Could you check a few things on this model? Use its own coordinates, in mm. A direction names the side the tool comes from. Coordinates: 2 decimals unless noted, no trailing zeros. Write each loop counter-clockwise with the first axis right and the second up, starting at its lowest first coordinate (ties: lowest second). Pieces come first, ordered by that corner, then holes.
```python
from build123d import *

# Parameters (mm, degrees)
ESBO_O1_R                = 9
ESBO_O1_R_2              = 6.15
RESSALTO_EXTRUS_O1_DEPTH = 38.8
ESBO_O1_2_R              = 6.15
RESSALTO_EXTRUS_O2_DEPTH = 41.8
ESBO_O2_R                = 1.5
CORTE_EXTRUS_O1_DEPTH    = 44.694850955


with BuildPart() as part:
    # Esbo_o1 → Ressalto-extrus_o1 (new body)
    with BuildSketch(Plane(origin=(0, 0, 0), x_dir=(1, 0, 0), z_dir=(0, 1, 0))):
        with Locations(Location((0, 0, 0), (0, 0, 270))):
            Circle(ESBO_O1_R)
        with Locations(Location((0, 0, 0), (0, 0, 270))):
            Circle(ESBO_O1_R_2, mode=Mode.SUBTRACT)
    extrude(amount=RESSALTO_EXTRUS_O1_DEPTH)

    # Esbo_o1_2 → Ressalto-extrus_o2 (add)
    with BuildSketch(Plane(origin=(0, 0, 0), x_dir=(1, 0, 0), z_dir=(0, 1, 0))):
        with Locations(Location((0, 0, 0), (0, 0, 270))):
            Circle(ESBO_O1_2_R)
    extrude(amount=RESSALTO_EXTRUS_O2_DEPTH)

    # Esbo_o2 → Corte-extrus_o1 (cut, through all)
    with BuildSketch(Plane(origin=(0, 41.8, 0), x_dir=(1, 0, 0), z_dir=(0, 1, 0))):
        with Locations(Location((0, 0, 0), (0, 0, 270))):
            Circle(ESBO_O2_R)
    extrude(amount=-CORTE_EXTRUS_O1_DEPTH, mode=Mode.SUBTRACT)


solid = part.part
```
1. For pin 1 (1 mm diameter, centred on x = -2.5, y = 31.5, fed in from -Z); pin 2 (6 mm diameter, centred on x = 6.5, y = 30, fed in from -Z); pin 3 (1.8 mm diameter, centred on x = 0, z = 0, fed in from -Y); pin 4 (2 mm diameter, centred on x = 6.5, y = 31.5, fed in from +Z), each with a flat end and sliding along its axis, tell me the tip position at first contact or that it passes through.
Verdict:
pin 1: stops at z = -8.77
pin 2: stops at z = -8.29
pin 3: passes through
pin 4: stops at z = 7.12
2. Please list where these lines run through material, in increasing order: line 1 along X through (y, z) = (24.5, 0); line 2 along Y through (x, z) = (0.25, -8); line 3 along Z through (x, y) = (-1.25, 12).
Verdict:
line 1: x = -9 to -1.5, 1.5 to 9
line 2: y = 0 to 38.8
line 3: z = -8.91 to -0.83, 0.83 to 8.91
3. I want a section at A-A on z = 0. Please give me the cut outline in (x, y), plus the area to 3 significant figures.
Verdict:
outline: (-9, 0) - (-1.5, 0) - (-1.5, 41.8) - (-6.15, 41.8) - (-6.15, 38.8) - (-9, 38.8) - close; (1.5, 0) - (9, 0) - (9, 38.8) - (6.15, 38.8) - (6.15, 41.8) - (1.5, 41.8) - close
area: 610 mm2
4. If we mould it in two halves opening along X, with no side actions, what happens to faces 3 (the face through (0.45, 21.19, 1.43)), 4 (the face through (2.703, 19.128, 8.584)), 5 (the face through (-2, 0, 0))? For each: pulls with the +X half, pulls with the -X half, needs draft (parallel to the pull), parting line crosses it, or undercut.
Verdict:
face 3: undercut
face 4: parting line crosses it
face 5: needs draft
5. I want a section at B-B on x = 0. Please give me the cut outline in (y, z).
Verdict:
outline: (0, -9) - (38.8, -9) - (38.8, -6.15) - (41.8, -6.15) - (41.8, -1.5) - (0, -1.5) - close; (0, 1.5) - (41.8, 1.5) - (41.8, 6.15) - (38.8, 6.15) - (38.8, 9) - (0, 9) - close
6. I want a section at C-C on y = 28. Please give me the cut outline in (x, z).
Verdict:
outline: circle Ø18 at (0, 0); hole circle Ø3 at (0, 0)
7. I want a section at D-D on x = -2.5. Please give me the cut outline in (y, z).
Verdict:
outline: (0, -8.65) - (38.8, -8.65) - (38.8, -5.62) - (41.8, -5.62) - (41.8, 5.62) - (38.8, 5.62) - (38.8, 8.65) - (0, 8.65) - close
8. On a 3-axis mill with a long thin cutter (end or side, diameter ignored), from which of +Z, -Z, +X, -X, +Y, -Y can I reach the whole of each face in a straight line? I mean faces 1 (the face through (-1.3, 41.8, 1.3)), 2 (the face through (-6.004, 40.279, -1.333)). Say none if no direction works.
Verdict:
face 1: +Z, -Z, +X, -X, +Y
face 2: +Y
